Work out the finished part from the listing and answer in its coordinate system (mm). A direction names the side the tool comes from. Round coordinates to 2 decimals unless told otherwise and drop trailing zeros. Loops run counter-clockwise (first coordinate to the right, second up) from the corner with the lowest first, then second, coordinate; pieces in that order, holes last.
```python
from build123d import *

# Parameters (mm, degrees)
BOSS_EXTRUDE1_DEPTH = 44
SKETCH2_R           = 1.25
CUT_EXTRUDE1_DEPTH  = 5
SKETCH3_R           = 1.25
CUT_EXTRUDE2_DEPTH  = 5


with BuildPart() as part:
    # Sketch1 → Boss-Extrude1 (new body)
    with BuildSketch(Plane.XY):
        Polygon((0, -4.041451884), (3.5, -2.020725942), (3.5, 2.020725942), (0, 4.041451884), (-3.5, 2.020725942), (-3.5, -2.020725942), align=None)
    extrude(amount=BOSS_EXTRUDE1_DEPTH)

    # Sketch2 → Cut-Extrude1 (cut)
    with BuildSketch(Plane.XY.offset(44)):
        Circle(SKETCH2_R)
    extrude(amount=-CUT_EXTRUDE1_DEPTH, mode=Mode.SUBTRACT)

    # Sketch3 → Cut-Extrude2 (cut)
    with BuildSketch(Plane(origin=(0, 0, 0), x_dir=(-1, 0, 0), z_dir=(0, 0, -1))):
        Circle(SKETCH3_R)
    extrude(amount=-CUT_EXTRUDE2_DEPTH, mode=Mode.SUBTRACT)


solid = part.part
```
1. Determine the mould class of faces 4 (the face through (0, 0, 5)), 5 (the face through (-1.8, -3, 21.7)), 6 (the face through (-1, 1, 44)), 7 (the face through (1.726, -3.045, 21.692)) for opening direction X: +X half, -X half, draft (parallel to the pull), parting line (faces both ways), or undercut.
Answer key:
face 4: undercut
face 5: -X half
face 6: draft
face 7: +X half
2. Find section D-D (y = -3.5). Write down the section's boundary in (x, z), then the cut area to 3 significant figures.
Answer key:
outline: (-0.94, 0) - (0.94, 0) - (0.94, 44) - (-0.94, 44) - close
area: 82.5 mm2
3. Find section A-A (y = 0). Write down the section's boundary in (x, z), then the cut area to 3 significant figures.
Answer key:
outline: (-3.5, 0) - (-1.25, 0) - (-1.25, 5) - (1.25, 5) - (1.25, 0) - (3.5, 0) - (3.5, 44) - (1.25, 44) - (1.25, 39) - (-1.25, 39) - (-1.25, 44) - (-3.5, 44) - close
area: 283 mm2
4. Find section B-B (z = 15). Write down the section's boundary in (x, y).
Answer key:
outline: (-3.5, -2.02) - (0, -4.04) - (3.5, -2.02) - (3.5, 2.02) - (0, 4.04) - (-3.5, 2.02) - close
5. Given pin 1 (1 mm diameter, centred on x = -0.5, y = 0, fed in from +Z); pin 2 (2 mm diameter, centred on x = 0, y = 0, fed in from -Z); pin 3 (1.5 mm diameter, centred on x = -2.5, z = 12, fed in from -Y), each flat-ended and moving along its own axis, determine where each tip first touches the part or whether it passes through.
Answer key:
pin 1: stops at z = 39
pin 2: stops at z = 5
pin 3: stops at y = -3.03
6. Find section C-C (x = -2.25). Write down the section's boundary in (y, z), then the cut area to 3 significant figures.
Answer key:
outline: (-2.74, 0) - (2.74, 0) - (2.74, 44) - (-2.74, 44) - close
area: 241 mm2
7. Consider probe 1 along Y at (x, z) = (0, 2.35); probe 2 along Z at (x, y) = (-0.5, -0.75); probe 3 along Y at (x, z) = (-1, 4). Determine where each line is inside the solid, lowest interval first.
Answer key:
probe 1: y = -4.04 to -1.25, 1.25 to 4.04
probe 2: z = 5 to 39
probe 3: y = -3.46 to -0.75, 0.75 to 3.46
8. Which of the six approach directions +Z, -Z, +X, -X, +Y, -Y give full straight-line access (tool end or side, diameter ignored) to faces 1 (the face through (-0.27, -1.22, 41.54)), 2 (the face through (0.27, -1.22, 2.46)), 3 (the face through (-1.726, 3.045, 21.692))?
Answer key:
face 1: +Z
face 2: -Z
face 3: +Z, -Z, -X, +Y
